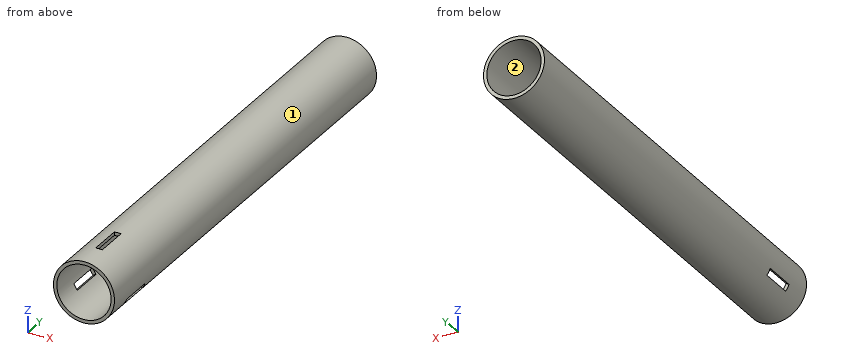
```python
from build123d import *

# Parameters (mm, degrees)
SKETCH1_R           = 45
SKETCH1_R_2         = 40
BOSS_EXTRUDE2_DEPTH = 700
SKETCH2_W           = 10
SKETCH2_H           = 50
CUT_EXTRUDE4_DEPTH  = 62
CIRPATTERN1_COUNT   = 3


with BuildPart() as part:
    # Sketch1 → Boss-Extrude2 (new body)
    with BuildSketch(Plane(origin=(0, 0, 0), x_dir=(1, 0, 0), z_dir=(0, 1, 0))):
        with Locations(Location((0, 0, 0), (0, 0, 270))):
            Circle(SKETCH1_R)
        with Locations(Location((0, 0, 0), (0, 0, 270))):
            Circle(SKETCH1_R_2, mode=Mode.SUBTRACT)
    extrude(amount=BOSS_EXTRUDE2_DEPTH)

    # Sketch2 → Cut-Extrude4 (cut)
    with BuildSketch(Plane.XY):
        with Locations((0, 65)):
            Rectangle(SKETCH2_W, SKETCH2_H)
    cut_extrude4 = extrude(amount=CUT_EXTRUDE4_DEPTH, mode=Mode.SUBTRACT)

    # CirPattern1: Cut-Extrude4 ×3 about axis
    cirpattern1_axis = Axis((0, 0, 0), (0, 1, 0))
    for i in range(1, CIRPATTERN1_COUNT):
        add(cut_extrude4.rotate(cirpattern1_axis, i * 360 / CIRPATTERN1_COUNT), mode=Mode.SUBTRACT)


solid = part.part
```
Could you check a few things on this model? Use its own coordinates, in mm. Face numbers are marked on the shaded views. Give positions to 0.01 mm unless a question says otherwise; leave off trailing zeros. Loops run counter-clockwise (first coordinate to the right, second up) from the corner with the lowest first, then second, coordinate; pieces in that order, holes last. Notation, with made-up numbers: (11, 71) - (54, 71) arc R11 ccw to (54, 80) - close; hole circle Ø5 at (63, -25.75). An arc over 180 degrees is marked (long way). Answer in a Markdown table with one row per item. Add a question column.
Q1. If we section it at A-A (y = 48): List the corners of the cut face in (x, z) for me.
Q2. Please list where these lines run through material, in increasing order: L1, parallel to X at y = 151, z = 0; L2, parallel to X at y = 93, z = -7; L3, parallel to Z at x = -10.5, y = 90.5. Write a range as from..to.
Q3. If we section it at D-D (y = 205): List the corners of the cut face in (x, z) for me.
Q4. We'd pull the mould along X, two halves only. Please class the marked faces 1 and 2: +X half, -X half, draft (parallel to the pull), parting line (faces both ways), or undercut.
Q5. If we section it at B-B (x = -21): List the corners of the cut face in (y, z) for me.
Q6. If we section it at C-C (z = 0): List the corners of the cut face in (x, y) for me.
Q7. For pin 1 (12 mm diameter, centred on x = -8, y = 205.5, fed in from +Z); pin 2 (1.5 mm diameter, centred on y = 65, z = 42, fed in from +X); pin 3 (7.5 mm diameter, centred on x = -38, z = -20.5, fed in from -Y); pin 4 (1 mm diameter, centred on y = 321, z = -35.5, fed in from -X), each with a flat end and sliding along its axis, tell me the tip position at first contact or that it passes through.
The answers:
| question | item | result |
|---|---|---|
| 1 | outline | (-41.23, -18.03) - (-36.87, -15.51) arc R40 cw to (-5, 39.69) - (-5, 44.72) arc R45 ccw to start; (-36.23, -26.69) arc R45 ccw to (36.23, -26.69) - (31.87, -24.17) arc R40 cw to (-31.87, -24.17) - close; (5, 39.69) arc R40 cw to (36.87, -15.51) - (41.23, -18.03) arc R45 ccw to (5, 44.72) - close |
| 2 | L1 | x = -45..-40, 40..45 |
| 2 | L2 | x = -44.45..-39.38, 39.38..44.45 |
| 2 | L3 | z = -43.76..-38.6, 38.6..43.76 |
| 3 | outline | circle Ø90 at (0, 0); hole circle Ø80 at (0, 0) |
| 4 | face 1 | parting line |
| 4 | face 2 | undercut |
| 5 | outline | (0, -39.8) - (700, -39.8) - (700, -34.04) - (0, -34.04) - close; (0, 34.04) - (700, 34.04) - (700, 39.8) - (0, 39.8) - close |
| 6 | outline | (-45, 0) - (-40, 0) - (-40, 700) - (-45, 700) - close; (40, 0) - (45, 0) - (45, 700) - (40, 700) - close |
| 7 | pin 1 | stops at z = 44.96 |
| 7 | pin 2 | stops at x = 17.98 |
| 7 | pin 3 | stops at y = 0 |
| 7 | pin 4 | stops at x = -28.28 |
